Check sheet for the modelled part. Datum: model origin and axes. Units: mm. Face numbers are marked on the shaded views. A direction names the side the tool comes from. Coordinates: 2 decimals unless noted, no trailing zeros. Write each loop counter-clockwise with the first axis right and the second up, starting at its lowest first coordinate (ties: lowest second). Pieces come first, ordered by that corner, then holes. Notation, with made-up numbers: (52.5, -2.75) -> (62.5, -2.75) arc R10 ccw to (62.5, 6.25) -> close; hole circle Ø8 at (-34, 68). An arc over 180 degrees is marked (long way). Put each result on its own line as item: value.
```python
from build123d import *

# Parameters (mm, degrees)
BOSS_EXTRUDE1_DEPTH     = 3
CUT_EXTRUDE1_DEPTH      = 32.176914536
CUT_EXTRUDE1_DEPTH_BACK = 32.176914536
SKETCH10_R              = 3.5
SKETCH11_R              = 1.5
CUT_EXTRUDE2_DEPTH      = 20


with BuildPart() as part:
    # Sketch1 → Boss-Extrude1 (new, symmetric)
    with BuildSketch(Plane.XY):
        with BuildLine():
            Line((5.196152423, -3), (30, -3))
            Line((30, -3), (30, 3))
            Line((30, 3), (5.196152423, 3))
            ThreePointArc((5.196152423, 3), (-6, 0), (5.196152423, -3))
        make_face()
    extrude(amount=BOSS_EXTRUDE1_DEPTH, both=True)

    # Sketch10 → Cut-Extrude1 (cut, two sides: drawn at the far end of the back side and taken through both)
    with BuildSketch(Plane.XY.offset(3).offset(-CUT_EXTRUDE1_DEPTH_BACK)):
        Circle(SKETCH10_R)
    extrude(amount=CUT_EXTRUDE1_DEPTH + CUT_EXTRUDE1_DEPTH_BACK, mode=Mode.SUBTRACT)

    # Sketch11 → Cut-Extrude2 (cut)
    with BuildSketch(Plane(origin=(30, 0, 0), x_dir=(0, 0, -1), z_dir=(1, 0, 0))):
        Circle(SKETCH11_R)
    extrude(amount=-CUT_EXTRUDE2_DEPTH, mode=Mode.SUBTRACT)


solid = part.part
```
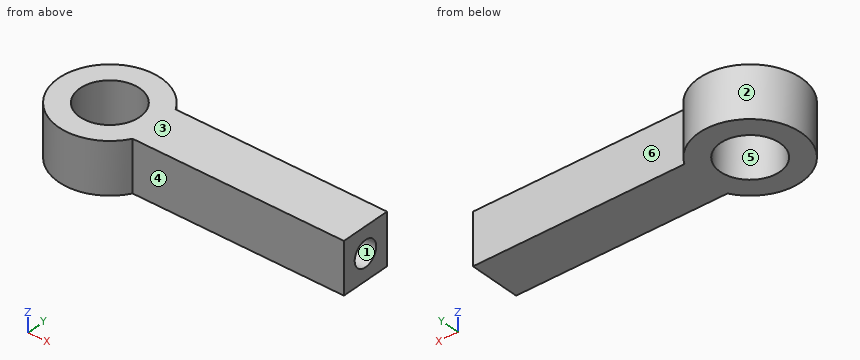
Q1. Mould release check, pull along Z, two halves, no side actions. Record for the marked faces 1, 2 and 3: released by +Z, released by -Z, zero draft, split by the parting line, or undercut.
Recorded:
face 1: undercut
face 2: zero draft
face 3: released by +Z
Q2. Depth check by flat-ended pin: P1, Ø1.5, axis at y = 0.5, z = 0.5, coming from the -X side; P2, Ø2.5, axis at y = 0, z = 0, coming from the +X side; P3, Ø3, axis at x = 16, z = -1.5, coming from the +Y side; P4, Ø1.8, axis at x = 18, z = 1.5, coming from the -Y side. Enter the tip coordinate at first touch or a pass-through.
Recorded:
P1: stops at x = -6
P2: stops at x = 10
P3: stops at y = 3
P4: stops at y = -3
Q3. Cross-section at C-C (z = 1.95). Record the cut outline in (x, y), plus the area to 3 significant figures.
Recorded:
outline: (5.2, -3) -> (30, -3) -> (30, 3) -> (5.2, 3) arc R6 ccw (long way) to start; hole circle Ø7 at (0, 0)
area: 220 mm2
Q4. Cross-section at A-A (x = 0). Record the cut outline in (y, z), plus the area to 3 significant figures.
Recorded:
outline: (-6, -3) -> (-3.5, -3) -> (-3.5, 3) -> (-6, 3) -> close; (3.5, -3) -> (6, -3) -> (6, 3) -> (3.5, 3) -> close
area: 30.0 mm2
Q5. Tool access check on the marked faces 4, 5 and 6. Record the directions out of +Z, -Z, +X, -X, +Y, -Y that give a thin tool (end or side, any length) a straight path to the whole face; none if there is none.
Recorded:
face 4: +Z, -Z, +X, -Y
face 5: +Z, -Z
face 6: +Z, -Z, +X, +Y
Q6. Material ranges on line 1 along Y through (x, z) = (20, 0); line 2 along Y through (x, z) = (7, -0.05); line 3 along X through (y, z) = (0, -0.75), recorded low to high.
Recorded:
line 1: y = -3 to -1.5, 1.5 to 3
line 2: y = -3 to 3
line 3: x = -6 to -3.5, 3.5 to 10
Q7. Cross-section at D-D (x = 18.5). Record the cut outline in (y, z).
Recorded:
outline: (-3, -3) -> (3, -3) -> (3, 3) -> (-3, 3) -> close; hole circle Ø3 at (0, 0)
Q8. Cross-section at B-B (y = 0). Record the cut outline in (x, z), plus the area to 3 significant figures.
Recorded:
outline: (-6, -3) -> (-3.5, -3) -> (-3.5, 3) -> (-6, 3) -> close; (3.5, -3) -> (30, -3) -> (30, -1.5) -> (10, -1.5) -> (10, 1.5) -> (30, 1.5) -> (30, 3) -> (3.5, 3) -> close
area: 114 mm2
